```python
from build123d import *

# Parameters (mm, degrees)
F3_R     = 60
F6_DEPTH = 250
F2_W     = 50
F2_H     = 300
F7_DEPTH = 625
F0_W     = 150
F0_H     = 40
F8_DEPTH = 75
F1_R     = 25
F9_DEPTH = 35


with BuildPart() as f5:
    # F4 (on Front) → F5 (revolve)
    with BuildSketch(Plane.XZ):
        with BuildLine():
            Line((470, 125), (82.91562, 125))
            ThreePointArc((82.91562, 125), (-70.931858, 132.169102), (-150, 0))
            Line((-150, 0), (950, 0))
            Line((950, 0), (950, 75))
            Line((950, 75), (650, 75))
            Line((650, 75), (470, 125))
        make_face()
    revolve(axis=Axis((400, 0, 0), (1, 0, 0)))

    # F3 (on Front) → F6 (cut, symmetric)
    with BuildSketch(Plane.XZ):
        Circle(F3_R)
    extrude(amount=F6_DEPTH, both=True, mode=Mode.SUBTRACT)

    # F2 (on Right) → F7 (cut, symmetric)
    with BuildSketch(Plane.YZ):
        with Locations((-125, 0)):
            Rectangle(F2_W, F2_H)
        with Locations((125, 0)):
            Rectangle(F2_W, F2_H)
    extrude(amount=F7_DEPTH, both=True, mode=Mode.SUBTRACT)

    # F0 (on Front) → F8 (cut, symmetric)
    with BuildSketch(Plane.XZ):
        with Locations((875, 55)):
            Rectangle(F0_W, F0_H)
        with Locations((875, -55)):
            Rectangle(F0_W, F0_H)
    extrude(amount=F8_DEPTH, both=True, mode=Mode.SUBTRACT)

    # F1 (on Top) → F9 (cut, symmetric)
    with BuildSketch(Plane.XY):
        with Locations((875, 0)):
            Circle(F1_R)
    extrude(amount=F9_DEPTH, both=True, mode=Mode.SUBTRACT)


solid = f5.part
```
Model file for the job. Use its own axes, mm. A direction names the side the tool comes from. Coordinates: 2 decimals unless noted, no trailing zeros. Loops run counter-clockwise (first coordinate to the right, second up) from the corner with the lowest first, then second, coordinate; pieces in that order, holes last. Notation, with made-up numbers: (-4, 17.25) - (25, 17.25) arc R6 ccw to (25, 28.25) - close; hole circle Ø2 at (-17.75, 25.5). An arc over 180 degrees is marked (long way). Answer as a JSON object with one key per item and string values. Group by question number.
(1) Cut at C-C (x = 875). Give the cut face in (y, z).
(2) Probe line 1 along Z through (x, y) = (0, 1); line 2 along Y through (x, z) = (875, 3); line 3 along X through (y, z) = (28.5, 8). List the from-to ranges inside material, lowest first.
(3) Cut at A-A (y = 0). Give the cut face in (x, z), then the cut area to 3 significant figures.
(4) Tool access for faces 1 (the face through (874, 30, 35)), 2 (the face through (273.75, 1.62, 124.99)), 3 (the face through (800, -1, -51)): list every direction of +Z, -Z, +X, -X, +Y, -Y with a clear straight run to the whole face (end or side of a thin tool).
(5) Cut at B-B (z = 0). Give the cut face in (x, y).
(6) Two-plate mould, pull along X, no slides. Class faces 4 (the face through (219, -100, -2)), 5 (the face through (-59.94, -1.4, 2.64)), 6 (the face through (950, -1, 0)): released by +X, released by -X, zero draft, split by the parting line, or undercut.
(7) Cut at D-D (x = 0). Give the cut face in (y, z).
(8) Flat gauge pins, fed straight in: pin 1 (10 mm diameter, centred on y = -55, z = -28.5, fed in from -X); pin 2 (2 mm diameter, centred on y = 48.5, z = 40, fed in from +X); pin 3 (2 mm diameter, centred on x = 463, z = 95, fed in from -Y). Where does each tip first touch, or does it go through?
Geometry says:
{
 "1": {"outline": "(-66.33, -35) - (-25, -35) - (-25, 35) - (-66.33, 35) arc R75 ccw to start; (25, -35) - (66.33, -35) arc R75 ccw to (66.33, 35) - (25, 35) - close"},
 "2": {"line 1": "z = -150 to -60, 60 to 150", "line 2": "y = -74.94 to -25, 25 to 74.94", "line 3": "x = -147.05 to -59.46, 59.46 to 950"},
 "3": {"outline": "(82.92, -125) - (470, -125) - (650, -75) - (800, -75) - (800, -35) - (850, -35) - (850, 35) - (800, 35) - (800, 75) - (650, 75) - (470, 125) - (82.92, 125) arc R150 ccw (long way) to start; (900, -35) - (950, -35) - (950, 35) - (900, 35) - close; hole circle Ø120 at (0, 0)", "area": "210,000 mm^2"},
 "4": {"face 1": "+Z, +X, +Y, -Y", "face 2": "+Z, +X", "face 3": "-Z, +X, +Y, -Y"},
 "5": {"outline": "(-111.8, -100) - (-60, -100) - (-60, 100) - (-111.8, 100) arc R150 ccw to start; (60, -100) - (560, -100) - (650, -75) - (950, -75) - (950, 75) - (650, 75) - (560, 100) - (60, 100) - close; hole circle Ø50 at (875, 0)"},
 "6": {"face 4": "zero draft", "face 5": "undercut", "face 6": "released by +X"},
 "7": {"outline": "(-100, -111.8) arc R150 ccw to (100, -111.8) - (100, -60) - (-100, -60) - close; (-100, 60) - (100, 60) - (100, 111.8) arc R150 ccw to (-100, 111.8) - close"},
 "8": {"pin 1": "stops at x = -138.77", "pin 2": "stops at x = 800", "pin 3": "stops at y = -82.4"}
}
